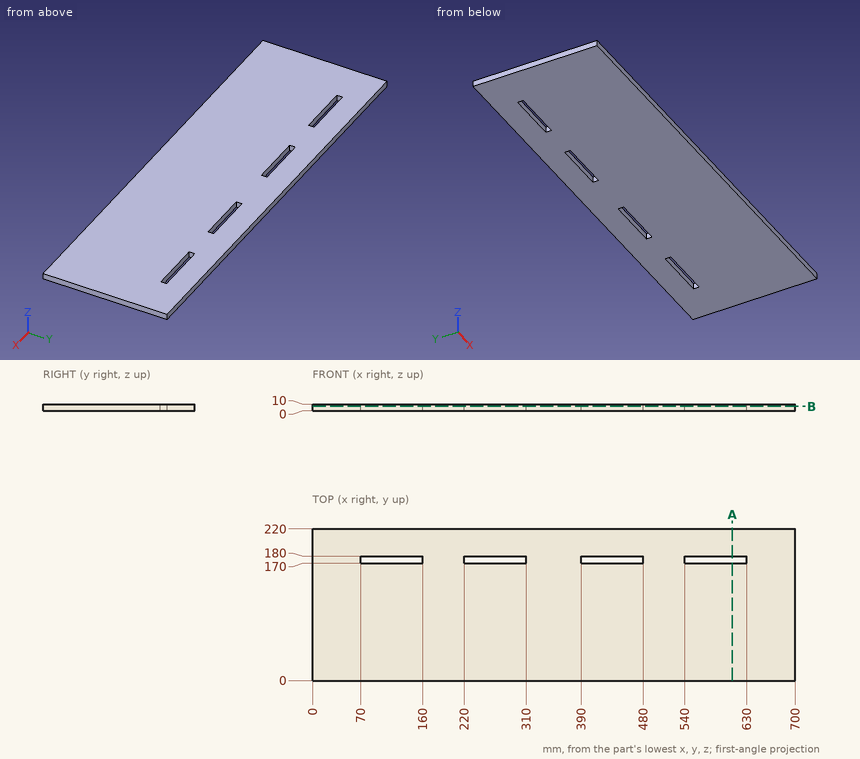
Print and shaded views of the part. All mm, measured from the part's lowest x, y and z. Round coordinates to 2 decimals unless told otherwise and drop trailing zeros. Write each loop counter-clockwise with the first axis right and the second up, starting at its lowest first coordinate (ties: lowest second). Pieces come first, ordered by that corner, then holes.
(1) Probe line 1 along Y through (x, z) = (78.5, 3.25). List the from-to ranges inside material, lowest first.
(2) Slice it at B-B, the plane z = 6.5. Write the cut outline in (x, y), and give its area (3 significant figures).
(3) Drop a flat-ended pin along its axis: P1, Ø3, axis at x = 271.5, z = 4.5, coming from the -Y side. Give the stop position or say it passes through.
(4) Slice it at A-A, the plane x = 609. Write the cut outline in (y, z), and give its area (3 significant figures).
From the geometry:
1. line 1: y = 0 to 170, 180 to 220
2. outline: (0, 0) - (700, 0) - (700, 220) - (0, 220) - close; hole (70, 170) - (160, 170) - (160, 180) - (70, 180) - close; hole (220, 170) - (310, 170) - (310, 180) - (220, 180) - close; hole (390, 170) - (480, 170) - (480, 180) - (390, 180) - close; hole (540, 170) - (630, 170) - (630, 180) - (540, 180) - close
2. area: 150,000 mm2
3. P1: stops at y = 0
4. outline: (0, 0) - (170, 0) - (170, 10) - (0, 10) - close; (180, 0) - (220, 0) - (220, 10) - (180, 10) - close
4. area: 2,100 mm2
